Can you work these out from the model? Positions are in its coordinate system, mm. A direction names the side the tool comes from. Give positions to 0.01 mm unless a question says otherwise; leave off trailing zeros. Order: outer loops, then holes, each group sorted by start corner. A loop starts at its lowest first (then second) coordinate and runs counter-clockwise, first axis right, second up. Notation, with made-up numbers: M 40.5,2.5 L 91.5,2.5 A5 cw 91.5,11.5 Z; hole C 31.25,5 d4. An arc over 180 degrees is marked long. One line per question, with ' | ' between items. Start each with the question number.
1) Please list where these lines run through material, in increasing order: line 1 along Z through (x, y) = (-1.75, 3.95); line 2 along X through (y, z) = (1.7, 55.5); line 3 along Z through (x, y) = (-7.5, 4.45). Write a range as [from, to].
2) If we section it at B-B, the plane z = -112: Please give me the cut outline in (x, y).
3) Thinking about a two-plate mould opening in Z: for faces 1 (the flat face through (0, 2, 131.5)), 2 (the flat face through (-5, 0, -2)), 3 (the flat face through (0, 2, 135.5)), which applies, +Z half, -Z half, draft (parallel to the pull), parting line (faces both ways), or undercut?
4) If we section it at A-A, the plane x = -0.5: Please give me the cut outline in (y, z), plus the area to 3 significant figures.
5) For faces 4 (the flat face through (4, 2, 2)), 5 (the flat face through (0, 2, -135.5)), which set-ups out of +Z, -Z, +X, -X, +Y, -Y let a thin tool reach every point of the face, with its end or its side?
6) If we section it at C-C, the plane y = 2.55: Please give me the cut outline in (x, z), plus the area to 3 significant figures.
```python
from build123d import *

# Parameters (mm, degrees)
SKETCH1_W           = 16
SKETCH1_H           = 271
SKETCH1_W_2         = 8
SKETCH1_H_2         = 263
BOSS_EXTRUDE1_DEPTH = 5
FILLET1_R           = 1.5


with BuildPart() as part:
    # Sketch1 → Boss-Extrude1 (new body)
    with BuildSketch(Plane(origin=(0, 0, 0), x_dir=(1, 0, 0), z_dir=(0, 1, 0))):
        Rectangle(SKETCH1_W, SKETCH1_H)
        Rectangle(SKETCH1_W_2, SKETCH1_H_2, mode=Mode.SUBTRACT)
    extrude(amount=BOSS_EXTRUDE1_DEPTH)

    # Fillet1
    fillet1_edges = [part.edges().sort_by_distance(p)[0] for p in [
        (8, 2.5, 135.5),
        (-8, 2.5, 135.5),
        (-8, 2.5, -135.5),
        (8, 2.5, -135.5),
    ]]
    fillet(fillet1_edges, radius=FILLET1_R)


solid = part.part
```
Results found:
1) line 1: z = [-135.5, -131.5], [131.5, 135.5] | line 2: x = [-8, -4], [4, 8] | line 3: z = [-135.12, 135.12]
2) outline: M -8,0 L -4,0 L -4,5 L -8,5 Z; M 4,0 L 8,0 L 8,5 L 4,5 Z
3) face 1: undercut | face 2: draft | face 3: +Z half
4) outline: M 0,-135.5 L 5,-135.5 L 5,-131.5 L 0,-131.5 Z; M 0,131.5 L 5,131.5 L 5,135.5 L 0,135.5 Z | area: 40.0 mm²
5) face 4: +Y, -Y | face 5: -Z, +X, -X, +Y, -Y
6) outline: M -8,-134 A1.5 ccw -6.5,-135.5 L 6.5,-135.5 A1.5 ccw 8,-134 L 8,134 A1.5 ccw 6.5,135.5 L -6.5,135.5 A1.5 ccw -8,134 Z; hole M -4,-131.5 L 4,-131.5 L 4,131.5 L -4,131.5 Z | area: 2,230 mm²
